The model under review builds one solid part; all positions refer to its coordinate system, in mm. Face numbers are marked on the shaded views. A direction names the side the tool comes from. Coordinates: 2 decimals unless noted, no trailing zeros. Write each loop counter-clockwise with the first axis right and the second up, starting at its lowest first coordinate (ties: lowest second). Pieces come first, ordered by that corner, then holes.
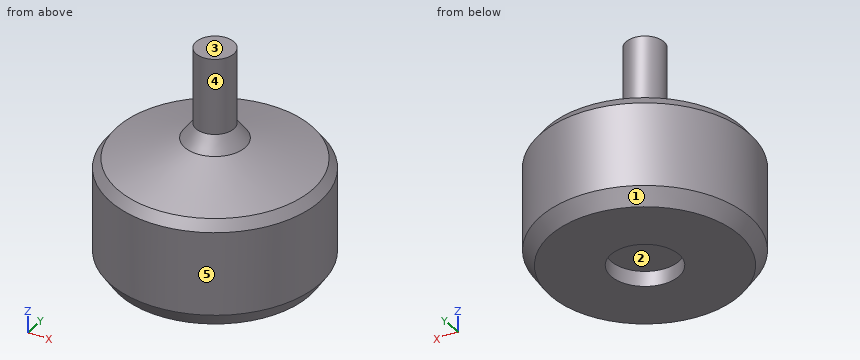
```python
from build123d import *

# Parameters (mm, degrees)
F5_R       = 12.5
F6_R       = 13.85
F11_FACE_R = 13.85
F7_R       = 13.85
F12_FACE_R = 13.85
F9_R       = 4
F13_FACE_R = 4
F8_R       = 2.5
F14_FACE_R = 2.5
F10_R      = 2.5
F16_SIZE   = 1
F17_R      = 4.5
F18_DEPTH  = 2


with BuildPart() as f11:
    # F5 (on Top) → F11 section 0
    with BuildSketch(Plane.XY):
        Circle(F5_R)
    # F6 (on offset) → F11 section 1
    with BuildSketch(Plane.XY.offset(2)):
        Circle(F6_R)
    loft()

    # F11_face (on face) → F12 section 0
    with BuildSketch(Plane.XY.offset(2)):
        Circle(F11_FACE_R)
    # F7 (on offset) → F12 section 1
    with BuildSketch(Plane.XY.offset(14)):
        Circle(F7_R)
    loft()

    # F12_face (on face) → F13 section 0
    with BuildSketch(Plane.XY.offset(14)):
        Circle(F12_FACE_R)
    # F9 (on offset) → F13 section 1
    with BuildSketch(Plane.XY.offset(17)):
        Circle(F9_R)
    loft()

    # F13_face (on face) → F14 section 0
    with BuildSketch(Plane.XY.offset(17)):
        Circle(F13_FACE_R)
    # F8 (on offset) → F14 section 1
    with BuildSketch(Plane.XY.offset(19)):
        Circle(F8_R)
    loft()

    # F14_face (on face) → F15 section 0
    with BuildSketch(Plane.XY.offset(19)):
        Circle(F14_FACE_R)
    # F10 (on offset) → F15 section 1
    with BuildSketch(Plane.XY.offset(29)):
        Circle(F10_R)
    loft()

    # F16
    f16_edges = [f11.edges().sort_by_distance(p)[0] for p in [
        (-13.85, 0, 14),
    ]]
    chamfer(f16_edges, length=F16_SIZE)

    # F17 (on Top) → F18 (cut)
    with BuildSketch(Plane.XY):
        Circle(F17_R)
    extrude(amount=F18_DEPTH, mode=Mode.SUBTRACT)


solid = f11.part
```
Item 1: Take a section at B-B, the plane z = 24.5. Write out the cut boundary in (x, y).
Solved:
outline: circle Ø5 at (0, 0)
Item 2: For pin 1 (12 mm diameter, centred on y = 10.5, z = 3.5, fed in from -X); pin 2 (10 mm diameter, centred on x = -8, z = 7.5, fed in from -Y); pin 3 (2 mm diameter, centred on x = -10, z = 13, fed in from -Y); pin 4 (10 mm diameter, centred on x = -1, y = 1, fed in from -Z), all flat-tipped, find the tip position at first contact; note any pin that passes through.
Solved:
pin 1: stops at x = -13.1
pin 2: stops at y = -13.52
pin 3: stops at y = -10.53
pin 4: stops at z = 0
Item 3: Take a section at A-A, the plane z = 9.5. Write out the cut boundary in (x, y).
Solved:
outline: circle Ø27.7 at (0, 0)
Item 4: To check wall thickness, follow line 1 along Y through (x, z) = (0, 0.6) (3 decimals); line 2 along Y through (x, z) = (0, 0.5); line 3 along Z through (x, y) = (5.25, -1.25). State the ranges of each line that lie inside material, in increasing order.
Solved:
line 1: y = -12.905 to -4.5, 4.5 to 12.905
line 2: y = -12.84 to -4.5, 4.5 to 12.84
line 3: z = 0 to 16.57
Item 5: Mouldability with a two-part tool opening along Y and no side actions: class the marked faces 1, 2 and 3 as pulls with the +Y half, pulls with the -Y half, needs draft (parallel to the pull), parting line crosses it, or undercut.
Solved:
face 1: parting line crosses it
face 2: undercut
face 3: needs draft
Item 6: Machinability: for the marked faces 4 and 5, which of the approach directions +Z, -Z, +X, -X, +Y, -Y give a long, thin tool a straight path to every point of the face, cutting with its end or side? Answer none if there is none.
Solved:
face 4: +Z
face 5: +Z, -Z
